Model file for the job. Use its own axes, mm. Face numbers are marked on the shaded views. A direction names the side the tool comes from. Give positions to 0.01 mm unless a question says otherwise; leave off trailing zeros. Loops run counter-clockwise (first coordinate to the right, second up) from the corner with the lowest first, then second, coordinate; pieces in that order, holes last. Notation, with made-up numbers: M -17,88 L -3,88 A22 cw -3,97 Z; hole C -29.5,-0.5 d3. An arc over 180 degrees is marked long. Answer in a Markdown table with one row per item.
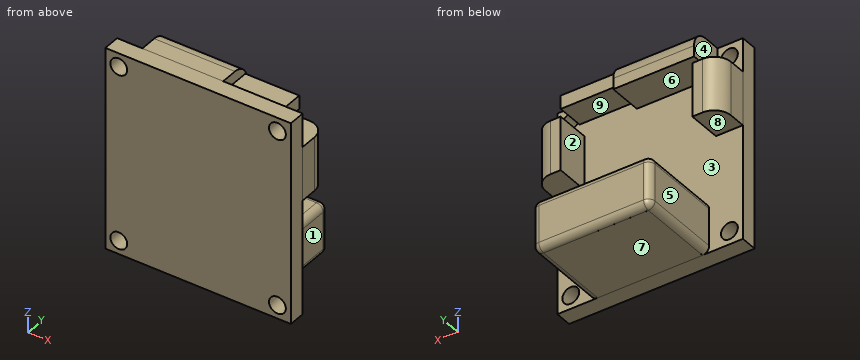
Autodesk Inventor part; units mm, degrees
ref_plane "YZ Plane" through (0, 0, 0) normal (1, 0, 0) x (0, 1, 0)
ref_plane "XZ Plane" through (0, 0, 0) normal (0, 1, 0) x (-1, 0, 0)
ref_plane "XY Plane" through (0, 0, 0) normal (0, 0, 1) x (1, 0, 0)
sketch "Boceto1" plane through (0, 0, 0) normal (0, 1, 0) x (-1, 0, 0)
  line L0 (27.559, 29.972) -> (-27.559, 29.972)
  line L1 (-27.559, 29.972) -> (-27.559, -29.972)
  line L2 (-27.559, -29.972) -> (27.559, -29.972)
  line L3 (27.559, -29.972) -> (27.559, 29.972)
  point P0 (0, 0)
  point P1 (0, -29.972)
  point P2 (0, 29.972)
  dimension "d0" = 59.944
  dimension "d1" = 55.118
  dimension "d44" = 29.972
  dimension "d45" = 27.559
extrude "Extrusión1" add sketch "Boceto1" along normal blind 5
sketch "Boceto2" plane through (0, 5, 0) normal (0, 1, 0) x (1, 0, 0)
  line L0 (27.559, 29.972) -> (-27.559, 29.972)
  line L1 (-17.559, 29.972) -> (17.559, 29.972)
  line L2 (17.559, 29.972) -> (17.559, 14.972)
  line L3 (17.559, 14.972) -> (-17.559, 14.972)
  line L4 (-17.559, 14.972) -> (-17.559, 29.972)
  line L5 (-27.559, 29.972) -> (-27.559, -29.972)
  line L6 (27.559, -29.972) -> (27.559, 29.972)
  point P0 (0, 0)
  point P1 (17.559, 22.472)
  point P2 (17.559, 29.972)
  dimension "d4" = 10
  dimension "d5" = 10
  dimension "d6" = 15
extrude "Extrusión2" add sketch "Boceto2" along normal blind 24.972
sketch "Boceto3" plane through (0, 5, 0) normal (0, 1, 0) x (1, 0, 0)
  line L0 (-27.559, -29.972) -> (27.559, -29.972)
  line L1 (-20.059, -29.972) -> (3.941, -29.972)
  line L2 (3.941, -29.972) -> (3.941, -21.7462)
  line L3 (3.941, -21.7462) -> (-20.059, -21.7462)
  line L4 (-20.059, -21.7462) -> (-20.059, -29.972)
  line L5 (-27.559, 29.972) -> (-27.559, -29.972)
  line L6 (-27.559, -19.972) -> (-19.559, -19.972)
  line L7 (-19.559, -19.972) -> (-19.559, -3.972)
  line L8 (-19.559, -3.972) -> (-27.559, -3.972)
  line L9 (-27.559, -3.972) -> (-27.559, -19.972)
  line L10 (27.559, -29.972) -> (27.559, 29.972)
  line L11 (27.559, -19.972) -> (19.559, -19.972)
  line L12 (19.559, -19.972) -> (19.559, -3.972)
  line L13 (19.559, -3.972) -> (27.559, -3.972)
  line L14 (27.559, -3.972) -> (27.559, -19.972)
  point P0 (0, 0)
  point P1 (-23.559, -19.972)
  point P2 (-20.059, -25.8591)
  point P3 (23.559, -19.972)
  point P4 (3.941, -29.972)
  dimension "d9" = 10
  dimension "d10" = 7.5
  dimension "d11" = 8
  dimension "d12" = 16
  dimension "d13" = 10
  dimension "d14" = 8
  dimension "d15" = 24
extrude "Extrusión3" add sketch "Boceto3" along normal blind 10
sketch "Boceto4" plane through (0, 5, 0) normal (0, 1, 0) x (1, 0, 0)
  line L0 (4.941, -23.972) -> (20.941, -23.972)
  line L1 (20.941, -23.972) -> (20.941, -27.972)
  line L2 (20.941, -27.972) -> (4.941, -27.972)
  line L3 (4.941, -27.972) -> (4.941, -23.972)
  line L4 (3.941, -29.972) -> (27.559, -29.972)
  line L5 (3.941, -29.972) -> (3.941, -21.7462)
  point P0 (0, 0)
  point P1 (20.941, -25.972)
  point P2 (4.941, -25.972)
  point P3 (3.941, -25.8591)
  dimension "d18" = 2
  dimension "d19" = 4
  dimension "d20" = 16
  dimension "d21" = 1
extrude "Extrusión4" add sketch "Boceto4" along normal blind 8
fillet "Empalme1" radius 2 1 edges at (0, 29.972, -14.972)
fillet "Empalme2" radius 2 3 edges at (-17.559, 16.486, -14.972) (-17.559, 29.3862, -15.5578) (-17.559, 29.972, -23.472)
fillet "Empalme3" radius 2 3 edges at (17.559, 16.486, -14.972) (17.559, 29.3862, -15.5578) (17.559, 29.972, -23.472)
fillet "Empalme4" radius 2 5 edges at (0, 29.972, -29.972) (-16.9732, 29.3862, -29.972) (-17.559, 16.486, -29.972) (16.9732, 29.3862, -29.972) (17.559, 16.486, -29.972)
fillet "Empalme5" radius 5 1 edges at (-27.559, 15, 11.972)
fillet "Empalme6" radius 5 1 edges at (-8.059, 15, 29.972)
fillet "Empalme7" radius 5 1 edges at (27.559, 15, 11.972)
sketch "Boceto6" plane through (27.559, 0, -29.972) normal (0, 0, -1) x (-1, 0, 0)
  line L0 (12, 27.972) -> (12, 5)
  line L1 (47.618, 5) -> (23.618, 5)
  line L2 (12, 27.972) -> (43.118, 27.972)
  line L3 (43.118, 27.972) -> (43.118, 5)
  line L4 (43.118, 5) -> (12, 5)
  line L5 (12, 5) -> (12, 27.972)
  line L6 (43.118, 27.972) -> (43.118, 5)
  point P0 (27.559, 0)
  point P1 (12, 5)
  dimension "d31" = 0
extrude "Extrusión5" add sketch "Boceto6" along normal blind 0.001
sketch "Boceto7" plane through (-27.559, 0, -29.972) normal (-1, 0, 0) x (0, 0, 1)
  line L0 (33.944, 5) -> (33.944, 15)
  line L1 (33.944, 5) -> (49.944, 5)
  line L2 (33.944, 10) -> (49.944, 10)
  line L3 (49.944, 10) -> (49.944, 5)
  line L4 (49.944, 5) -> (33.944, 5)
  line L5 (33.944, 5) -> (33.944, 10)
  point P0 (29.972, 0)
extrude "Extrusión6" add sketch "Boceto7" along normal blind 0.001
sketch "Boceto8" plane through (-27.559, 0, 29.972) normal (0, 0, 1) x (1, 0, 0)
  line L0 (7.5, 5) -> (7.5, 15)
  line L1 (43.118, 5) -> (12, 5)
  line L2 (7.5, 10) -> (31.5, 10)
  line L3 (31.5, 10) -> (31.5, 5)
  line L4 (31.5, 5) -> (7.5, 5)
  line L5 (7.5, 5) -> (7.5, 10)
  line L6 (31.5, 5) -> (31.5, 10)
  point P0 (27.559, 0)
  point P1 (12, 5)
  dimension "d36" = 0
extrude "Extrusión7" add sketch "Boceto8" along normal blind 0.001
sketch "Boceto9" plane through (27.559, 0, 29.972) normal (1, 0, 0) x (0, 0, -1)
  line L0 (10, 5) -> (10, 15)
  line L1 (26, 5) -> (10, 5)
  line L2 (10, 10) -> (26, 10)
  line L3 (26, 10) -> (26, 5)
  line L4 (26, 5) -> (10, 5)
  line L5 (10, 5) -> (10, 10)
  point P0 (29.972, 0)
extrude "Extrusión8" add sketch "Boceto9" along normal blind 0.001
sketch "Boceto10" plane through (0, 5, 0) normal (0, 1, 0) x (1, 0, 0)
  circle A0 centre (-23.559, 25.972) radius 2.5
  line L0 (-27.559, 29.972) -> (-27.559, -3.972)
  line L1 (-15.559, 29.972) -> (-27.559, 29.972)
  line L2 (0, 36.742) -> (0, -44.1649)
  line L3 (-51.3406, 0) -> (46.1301, 0)
  circle A1 centre (23.559, 25.972) radius 2.5
  circle A2 centre (-23.559, -25.972) radius 2.5
  line L4 (-27.559, -29.972) -> (-27.559, 3.972)
  circle A3 centre (23.559, -25.972) radius 2.5
  point P0 (0, 0)
  point P1 (27.559, 29.972)
  dimension "d41" = 5
  dimension "d42" = 4
  dimension "d43" = 4
extrude "Extrusión9" cut sketch "Boceto10" against normal blind 5
properties part number "Puente H"
Q1. Saw through at A-A (z = -20). Give the cut face in (x, y).
Reported:
| item | result |
|---|---|
| outline | M -27.56,0 L 27.56,0 L 27.56,5 L 17.56,5 L 17.56,27.97 A2 ccw 15.56,29.97 L -15.56,29.97 A2 ccw -17.56,27.97 L -17.56,5 L -27.56,5 Z |
Q2. Mould opens along X. For the marked faces 1, 2, 3 and 4 say: released by +X, released by -X, zero draft, split by the parting line, or undercut.
Reported:
| item | result |
|---|---|
| face 1 | released by +X |
| face 2 | undercut |
| face 3 | undercut |
| face 4 | released by -X |
Q3. Saw through at C-C (x = 24). Give the cut face in (y, z).
Reported:
| item | result |
|---|---|
| outline | M 0,-29.97 L 5,-29.97 L 5,-28.43 L 0,-28.43 Z; M 0,-23.51 L 5,-23.51 L 5,3.97 L 14.79,3.97 L 14.79,19.97 L 5,19.97 L 5,23.51 L 0,23.51 Z; M 0,28.43 L 5,28.43 L 5,29.97 L 0,29.97 Z |
Q4. Drop flat-ended pins along their axis: pin 1 (5 mm diameter, centred on x = 4.5, z = 11, fed in from +Y); pin 2 (6.5 mm diameter, centred on y = 10, z = 26.5, fed in from +X); pin 3 (1.2 mm diameter, centred on y = 9, z = 25.5, fed in from -X); pin 4 (12 mm diameter, centred on y = 18.5, z = -3, fed in from -X). Give the stop position or say it passes through.
Reported:
| item | result |
|---|---|
| pin 1 | y = 5 |
| pin 2 | x = 20.94 |
| pin 3 | x = -20.06 |
| pin 4 | through |
Q5. 3-axis set-ups, long thin cutter, end or side, ignore diameter. For the marked faces 5, 6, 7, 8 and 9: which of +Z, -Z, +X, -X, +Y, -Y reach the whole face in a straight line?
Reported:
| item | result |
|---|---|
| face 5 | -Z, -X, +Y |
| face 6 | +X, -X, +Y |
| face 7 | -Z, +X, -X, +Y, -Y |
| face 8 | -Z, +X, -X, +Y |
| face 9 | +X, +Y |
Q6. Saw through at B-B (y = 2.5). Give the cut face in (x, z), and give its area (3 significant figures).
Reported:
| item | result |
|---|---|
| outline | M -27.56,-29.97 L 27.56,-29.97 L 27.56,29.97 L -27.56,29.97 Z; hole C -23.56,-25.97 d5; hole C -23.56,25.97 d5; hole C 23.56,-25.97 d5; hole C 23.56,25.97 d5 |
| area | 3,230 mm² |
Q7. Probe probe 1 along Z at (x, y) = (-2, 8.75); probe 2 along X at (y, z) = (2, 25); probe 3 along Z at (x, y) = (23, 3.25). List the from-to ranges inside material, lowest first.
Reported:
| item | result |
|---|---|
| probe 1 | -29.97 to -14.97, 21.75 to 29.97 |
| probe 2 | -27.56 to -25.86, -21.26 to 21.26, 25.86 to 27.56 |
| probe 3 | -29.97 to -28.41, -23.54 to 23.54, 28.41 to 29.97 |
